from build123d import *

# Parameters (mm, degrees)
F0_W     = 60
F0_H     = 60
F1_DEPTH = 6
F2_T     = -2.5
F3_W     = 8
F3_H     = 22
F3_W_2   = 22
F3_H_2   = 8
F4_DEPTH = 6
F5_W     = 1.5
F5_H     = 22
F6_W     = 22
F6_H     = 1.5
F7_DEPTH = 6
F8_R     = 5


with BuildPart() as f1:
    # F0 (on Top) → F1 (new body)
    with BuildSketch(Plane.XY):
        with Locations((30, -30)):
            Rectangle(F0_W, F0_H)
    extrude(amount=F1_DEPTH)

    # F2
    f2_openings = [f1.faces().sort_by_distance(p)[0] for p in [
        (30, -30, 6),
    ]]
    offset(amount=F2_T, openings=f2_openings)

    # F3 (on face) → F4 (join)
    with BuildSketch(Plane.XY.offset(2.5)):
        with Locations((15, -25)):
            Rectangle(F3_W, F3_H)
        with Locations((35, -45.2)):
            Rectangle(F3_W_2, F3_H_2)
    extrude(amount=F4_DEPTH)

    # F5 (on face) + F6 (on face) → F7 (cut)
    with BuildSketch(Plane.XY.offset(8.5)):
        with Locations((15, -25)):
            Rectangle(F5_W, F5_H)
    with BuildSketch(Plane.XY.offset(8.5)):
        with Locations((35, -45.2)):
            Rectangle(F6_W, F6_H)
    extrude(amount=-F7_DEPTH, mode=Mode.SUBTRACT)

    # F8
    f8_edges = [f1.edges().sort_by_distance(p)[0] for p in [
        (30, -60, 0),
        (60, -30, 0),
        (0, -30, 0),
        (30, 0, 0),
    ]]
    fillet(f8_edges, radius=F8_R)


solid = f1.part
Read the model definition and answer for the solid it produces. Units are mm, in the model's axes. A direction names the side the tool comes from. Round coordinates to 2 decimals unless told otherwise and drop trailing zeros. Write each loop counter-clockwise with the first axis right and the second up, starting at its lowest first coordinate (ties: lowest second). Pieces come first, ordered by that corner, then holes.
Q1. The mould has two halves that part along X. Classify faces 1 (the face through (1, -30, 2)), 2 (the face through (2.5, -30, 4)), 3 (the face through (13, -25, 8.5)), 4 (the face through (13, -14, 5)): released by +X, released by -X, zero draft, split by the parting line, or undercut.
Values:
face 1: released by -X
face 2: undercut
face 3: zero draft
face 4: undercut
Q2. Find section A-A on x = 42. Determine the outline of the cut face in (y, z).
Values:
outline: (-60, 5) arc R5 ccw to (-55, 0) - (-5, 0) arc R5 ccw to (0, 5) - (0, 6) - (-2.5, 6) - (-2.5, 2.5) - (-41.2, 2.5) - (-41.2, 8.5) - (-44.45, 8.5) - (-44.45, 2.5) - (-45.95, 2.5) - (-45.95, 8.5) - (-49.2, 8.5) - (-49.2, 2.5) - (-57.5, 2.5) - (-57.5, 6) - (-60, 6) - close
Q3. Find section B-B on y = -12.5. Determine the outline of the cut face in (x, z).
Values:
outline: (0, 5) arc R5 ccw to (5, 0) - (55, 0) arc R5 ccw to (60, 5) - (60, 6) - (57.5, 6) - (57.5, 2.5) - (2.5, 2.5) - (2.5, 6) - (0, 6) - close
Q4. A tool of negligible diameter and unlimited length cuts with its end or side. For faces 5 (the face through (30, -59, 2)), 6 (the face through (17, -36, 5)), from which of +Z, -Z, +X, -X, +Y, -Y can it reach the whole face along a straight path? Write none if from no direction.
Values:
face 5: -Z, +X, -X, -Y
face 6: +Z
Q5. Flat-ended cylindrical pins translate along their axes: P1, Ø1.5, axis at x = 17, y = -52.5, coming from the +Z side; P2, Ø1.8, axis at x = 27.5, z = 3.5, coming from the +Y side; P3, Ø2, axis at x = 43.5, z = 1, coming from the -Y side. Find the tip coordinate at first contact, or state that the pin passes through.
Values:
P1: stops at z = 2.5
P2: stops at y = -0.04
P3: stops at y = -59
Q6. Find section D-D on y = -19. Determine the outline of the cut face in (x, z), and give its area (3 significant figures).
Values:
outline: (0, 5) arc R5 ccw to (5, 0) - (55, 0) arc R5 ccw to (60, 5) - (60, 6) - (57.5, 6) - (57.5, 2.5) - (19, 2.5) - (19, 8.5) - (15.75, 8.5) - (15.75, 2.5) - (14.25, 2.5) - (14.25, 8.5) - (11, 8.5) - (11, 2.5) - (2.5, 2.5) - (2.5, 6) - (0, 6) - close
area: 196 mm2
Q7. Straight lines are drawn through the part: line 1 (X direction, y = -23.5, z = 4.75); line 2 (Y direction, x = 26, z = 4.75); line 3 (Y direction, x = 35.5, z = 7.5). For each, find the intervals that lie inside material, in ascending order.
Values:
line 1: x = 0.01 to 2.5, 11 to 14.25, 15.75 to 19, 57.5 to 59.99
line 2: y = -59.99 to -57.5, -49.2 to -45.95, -44.45 to -41.2, -2.5 to -0.01
line 3: y = -49.2 to -45.95, -44.45 to -41.2
Q8. Find section C-C on x = 53. Determine the outline of the cut face in (y, z), and give its area (3 significant figures).
Values:
outline: (-60, 5) arc R5 ccw to (-55, 0) - (-5, 0) arc R5 ccw to (0, 5) - (0, 6) - (-2.5, 6) - (-2.5, 2.5) - (-57.5, 2.5) - (-57.5, 6) - (-60, 6) - close
area: 157 mm2
